```python
from build123d import *

# Parameters (mm, degrees)
SKETCH1_W           = 6.1
SKETCH1_H           = 5
BOSS_EXTRUDE1_DEPTH = 12.1
SKETCH2_R           = 2.8
BOSS_EXTRUDE2_DEPTH = 2
SKETCH3_R           = 1.8
CUT_EXTRUDE1_DEPTH  = 10
SKETCH4_R           = 0.75
BOSS_EXTRUDE3_DEPTH = 0.8
SKETCH5_W           = 0.6
SKETCH5_H           = 1.1
SKETCH5_H_2         = 0.1
SKETCH5_H_3         = 1.2
BOSS_EXTRUDE4_DEPTH = 3
FILLET1_R           = 0.5
FILLET2_R           = 0.1


with BuildPart() as part:
    # Sketch1 → Boss-Extrude1 (new body)
    with BuildSketch(Plane.XY):
        Rectangle(SKETCH1_W, SKETCH1_H)
    extrude(amount=BOSS_EXTRUDE1_DEPTH)

    # Sketch2 → Boss-Extrude2 (add)
    with BuildSketch(Plane.XY.offset(12.1)):
        with Locations(Location((0, 0, 0), (0, 0, 116.765500577))):
            Circle(SKETCH2_R)
    extrude(amount=BOSS_EXTRUDE2_DEPTH)

    # Sketch3 → Cut-Extrude1 (cut)
    with BuildSketch(Plane.XY.offset(14.1)):
        Circle(SKETCH3_R)
    extrude(amount=-CUT_EXTRUDE1_DEPTH, mode=Mode.SUBTRACT)

    # Sketch4 → Boss-Extrude3 (add)
    with BuildSketch(Plane.XZ.offset(2.5)):
        with Locations(Location((0, 10.5, 0), (0, 0, 90))):
            Circle(SKETCH4_R)
        with Locations(Location((0, 3.5, 0), (0, 0, 90))):
            Circle(SKETCH4_R)
    extrude(amount=BOSS_EXTRUDE3_DEPTH)

    # Sketch5 → Boss-Extrude4 (add)
    with BuildSketch(Plane.XZ.offset(2.5)):
        with Locations((-2.3, 1.95)):
            Rectangle(SKETCH5_W, SKETCH5_H)
        with Locations((-2.3, 1.35)):
            Rectangle(SKETCH5_W, SKETCH5_H_2)
        with Locations((-2.3, 5.9)):
            Rectangle(SKETCH5_W, SKETCH5_H_3)
        with Locations((2.3, 0.75)):
            Rectangle(SKETCH5_W, SKETCH5_H)
        with Locations((2.3, 1.35)):
            Rectangle(SKETCH5_W, SKETCH5_H_2)
        with Locations((-2.3, 8.9)):
            Rectangle(SKETCH5_W, SKETCH5_H_3)
    extrude(amount=BOSS_EXTRUDE4_DEPTH)

    # Fillet1
    fillet1_edges = [part.edges().sort_by_distance(p)[0] for p in [
        (-2.3, -5.5, 1.3),
        (-2.3, -5.5, 2.5),
        (-2.3, -5.5, 5.3),
        (-2.3, -5.5, 6.5),
        (2.3, -5.5, 0.2),
        (2.3, -5.5, 1.4),
        (-2.3, -5.5, 8.3),
        (-2.3, -5.5, 9.5),
    ]]
    fillet(fillet1_edges, radius=FILLET1_R)

    # Fillet2
    fillet2_edges = [part.edges().sort_by_distance(p)[0] for p in [
        (0, -3.3, 9.75),
        (0, -3.3, 2.75),
    ]]
    fillet(fillet2_edges, radius=FILLET2_R)


solid = part.part
```
Work out the finished part from the listing and answer in its coordinate system (mm). A direction names the side the tool comes from. Round coordinates to 2 decimals unless told otherwise and drop trailing zeros. Write each loop counter-clockwise with the first axis right and the second up, starting at its lowest first coordinate (ties: lowest second). Pieces come first, ordered by that corner, then holes.
1) A cutting plane is placed at C-C on z = 3.5. Determine the outline of the cut face in (x, y), and give its area (3 significant figures).
2) Which of the six approach directions +Z, -Z, +X, -X, +Y, -Y give full straight-line access (tool end or side, diameter ignored) to faces 1 (the face through (0, -2.5, 6)), 2 (the face through (-2.6, -4, 6)), 3 (the face through (-2, -4, 6))?
3) Consider probe 1 along Y at (x, z) = (0, 10); probe 2 along Y at (x, z) = (0, 7.75); probe 3 along Y at (x, z) = (-2.25, 4.5). Determine where each line is inside the solid, lowest interval first.
4) A cutting plane is placed at B-B on z = 10.5. Determine the outline of the cut face in (x, y), and give its area (3 significant figures).
5) A cutting plane is placed at D-D on y = -1.5. Determine the outline of the cut face in (x, z), and give its area (3 significant figures).
6) A cutting plane is placed at A-A on x = 0. Determine the outline of the cut face in (y, z).
7) Determine the mould class of faces 4 (the face through (0, -3.3, 3.5)), 5 (the face through (-2.6, -4, 2)), 6 (the face through (0, 0, 4.1)) for opening direction Y: pulls with the +Y half, pulls with the -Y half, needs draft (parallel to the pull), parting line crosses it, or undercut.
8) Flat-ended cylindrical pins translate along their axes: P1, Ø1, axis at y = -4.5, z = 6, coming from the +X side; P2, Ø1, axis at y = -4, z = 1, coming from the +X side; P3, Ø1, axis at y = -4, z = 9, coming from the -X side. Find the tip coordinate at first contact, or state that the pin passes through.
Entries:
1. outline: (-3.05, -2.5) - (-0.75, -2.5) - (-0.75, -3.2) arc R0.1 ccw to (-0.65, -3.3) - (0.65, -3.3) arc R0.1 ccw to (0.75, -3.2) - (0.75, -2.5) - (3.05, -2.5) - (3.05, 2.5) - (-3.05, 2.5) - close
1. area: 31.7 mm2
2. face 1: -Y
2. face 2: +Z, -Z, -X, -Y
2. face 3: +Z, -Z, +X, -Y
3. probe 1: y = -3.3 to -1.8, 1.8 to 2.5
3. probe 2: y = -2.5 to -1.8, 1.8 to 2.5
3. probe 3: y = -2.5 to 2.5
4. outline: (-3.05, -2.5) - (-0.75, -2.5) - (-0.75, -3.2) arc R0.1 ccw to (-0.65, -3.3) - (0.65, -3.3) arc R0.1 ccw to (0.75, -3.2) - (0.75, -2.5) - (3.05, -2.5) - (3.05, 2.5) - (-3.05, 2.5) - close; hole circle Ø3.6 at (0, 0)
4. area: 21.5 mm2
5. outline: (-3.05, 0) - (3.05, 0) - (3.05, 12.1) - (2.36, 12.1) - (2.36, 14.1) - (0.99, 14.1) - (0.99, 4.1) - (-0.99, 4.1) - (-0.99, 14.1) - (-2.36, 14.1) - (-2.36, 12.1) - (-3.05, 12.1) - close
5. area: 63.4 mm2
6. outline: (-3.3, 2.85) arc R0.1 ccw to (-3.2, 2.75) - (-2.5, 2.75) - (-2.5, 0) - (2.5, 0) - (2.5, 12.1) - (2.8, 12.1) - (2.8, 14.1) - (1.8, 14.1) - (1.8, 4.1) - (-1.8, 4.1) - (-1.8, 14.1) - (-2.8, 14.1) - (-2.8, 12.1) - (-2.5, 12.1) - (-2.5, 11.25) - (-3.2, 11.25) arc R0.1 ccw to (-3.3, 11.15) - (-3.3, 9.85) arc R0.1 ccw to (-3.2, 9.75) - (-2.5, 9.75) - (-2.5, 4.25) - (-3.2, 4.25) arc R0.1 ccw to (-3.3, 4.15) - close
7. face 4: pulls with the -Y half
7. face 5: needs draft
7. face 6: undercut
8. P1: stops at x = -2
8. P2: stops at x = 2.6
8. P3: stops at x = -2.6
